from build123d import *

# Parameters (mm, degrees)
EXTRUDE_1_DEPTH     = 4
CUT_EXTRUDE_1_DEPTH = 1.5
CUT_EXTRUDE_2_DEPTH = 6


with BuildPart() as part:
    # Эскиз1 → Бобышка-Вытянуть1 (new body, symmetric)
    with BuildSketch(Plane.XY):
        Polygon((4, 0), (-4, 0), (-4, -1.5), (-8, -1.5), (-8, -6.5), (8, -6.5), (8, -1.5), (4, -1.5), align=None)
    extrude(amount=EXTRUDE_1_DEPTH, both=True)

    # Эскиз3 → Отверстие обработанное метчиком M42 (revolve, cut)
    with BuildSketch(Plane(origin=(0, 0, 0), x_dir=(0, 0, 1), z_dir=(1, 0, 0))):
        Polygon((0, 0), (0, 6.5), (2.15, 6.5), (1.65, 6), (1.65, 0.5), (2.15, 0), align=None)
    revolve(axis=Axis((0, 6.35, 0), (0, -1, 0)), mode=Mode.SUBTRACT)

    # Эскиз4 → Вырез-Вытянуть1 (cut)
    with BuildSketch(Plane(origin=(0, 0, 0), x_dir=(1, 0, 0), z_dir=(0, 1, 0))):
        with BuildLine():
            Line((-4, 4), (-4, 0))
            ThreePointArc((-4, 0), (-2.828427125, 2.828427125), (0, 4))
            Line((0, 4), (-4, 4))
        make_face()
        with BuildLine():
            Line((0, -4), (4, -4))
            Line((4, -4), (4, 0))
            ThreePointArc((4, 0), (2.828427125, -2.828427125), (0, -4))
        make_face()
    extrude(amount=-CUT_EXTRUDE_1_DEPTH, mode=Mode.SUBTRACT)

    # Эскиз5 → Вырез-Вытянуть2 (cut, through all)
    with BuildSketch(Plane(origin=(0, -1.5, 0), x_dir=(1, 0, 0), z_dir=(0, 1, 0))):
        with BuildLine():
            Line((-8, 0), (-8, 4))
            Line((-8, 4), (-6.92820323, 4))
            ThreePointArc((-6.92820323, 4), (-7.72740661, 2.070552361), (-8, 0))
        make_face()
        with BuildLine():
            Line((8, 0), (8, -4))
            Line((8, -4), (6.92820323, -4))
            ThreePointArc((6.92820323, -4), (7.72740661, -2.070552361), (8, 0))
        make_face()
    extrude(amount=-CUT_EXTRUDE_2_DEPTH, mode=Mode.SUBTRACT)

    # Вырез-По траектории1: sweep along a path in Эскиз7
    with BuildLine(Plane.XZ.offset(6.5)) as sweep_1_path:
        Line((0, 8), (-8, 8))
        Line((-8, 8), (-8, 0))
        ThreePointArc((-8, 0), (-5.656854249, -5.656854249), (0, -8))
        Line((0, -8), (8, -8))
        Line((8, -8), (8, 0))
        ThreePointArc((8, 0), (5.656854249, 5.656854249), (0, 8))
    # Эскиз6 → Вырез-По траектории1 (sweep, cut)
    with BuildSketch(Plane.XY.offset(4)):
        Polygon((-8, -3), (-8, -6.5), (-4, -6.5), align=None)
    sweep(path=sweep_1_path.line, transition=Transition.RIGHT, mode=Mode.SUBTRACT)


solid = part.part
Read the model definition and answer for the solid it produces. Units are mm, in the model's axes. A direction names the side the tool comes from. Round coordinates to 2 decimals unless told otherwise and drop trailing zeros. Order: outer loops, then holes, each group sorted by start corner. A loop starts at its lowest first (then second) coordinate and runs counter-clockwise, first axis right, second up.
1) For faces 1 (the face through (-4, -1, 2)), 2 (the face through (2.859, -0.74, 2.797)), 3 (the face through (2, -6.5, -2)), 4 (the face through (-2.859, -0.74, -2.797)), 5 (the face through (4, -1, -2)), determine the directions among +Z, -Z, +X, -X, +Y, -Y from which every point of the face is accessible in a straight line to the end or side of a thin tool.
2) The part is cut by section A-A on y = -2. Write down the section's boundary in (x, z).
3) Straight lines are drawn through the part: L1, parallel to Z at x = 0, y = -1.6; L2, parallel to Z at x = -1.25, y = -1; L3, parallel to X at y = -4, z = 0. For each, find the intervals that lie inside material, in ascending order.
4) The mould has two halves that part along X. Classify faces 6 (the face through (-8, -2, 2)), 7 (the face through (5.086, -5.114, 2.304)), 8 (the face through (-1.115, -3.212, -1.216)): released by +X, released by -X, zero draft, split by the parting line, or undercut.
5) Flat-ended cylindrical pins translate along their axes: pin 1 (1.2 mm diameter, centred on y = -0.5, z = -2.5, fed in from +X); pin 2 (4 mm diameter, centred on x = 0, z = 0, fed in from -Y). Find the tip coordinate at first contact, or state that the pin passes through.
6) The part is cut by section B-B on y = -1. Write down the section's boundary in (x, z).
Resolved:
1. face 1: +Z, -Z, -X, +Y
1. face 2: +Z, +X, +Y
1. face 3: +Z, -Z, +X, -X, -Y
1. face 4: -Z, -X, +Y
1. face 5: +Z, -Z, +X, +Y
2. outline: (-8, 0) arc R8 ccw to (-6.93, -4) - (8, -4) - (8, 0) arc R8 ccw to (6.93, 4) - (-8, 4) - close; hole circle Ø3.3 at (0, 0)
3. L1: z = -4 to -1.65, 1.65 to 4
3. L2: z = -3.8 to -1.08, 1.08 to 4
3. L3: x = -6.86 to -1.65, 1.65 to 6.86
4. face 6: released by -X
4. face 7: released by +X
4. face 8: undercut
5. pin 1: stops at x = 4
5. pin 2: stops at y = -6.35
6. outline: (-4, 0) arc R4 ccw to (0, -4) - (4, -4) - (4, 0) arc R4 ccw to (0, 4) - (-4, 4) - close; hole circle Ø3.3 at (0, 0)
